from build123d import *

# Parameters (mm, degrees)
SKETCH_15_W          = 13
SKETCH_15_H          = 25
EXTRUDE_4_DEPTH      = 20
CUT_EXTRUDE_START    = 1
SKETCH_16_W          = 12
SKETCH_16_H          = 23
CUT_EXTRUDE_47_DEPTH = 24.6018292
CUT_EXTRUDE_48_DEPTH = 25.6018292


with BuildPart() as part:
    # 스케치15 → 보스-돌출4 (new body)
    with BuildSketch(Plane(origin=(0, 0, 0), x_dir=(1, 0, 0), z_dir=(0, 1, 0))):
        with Locations((0.5, 0)):
            Rectangle(SKETCH_15_W, SKETCH_15_H)
    extrude(amount=EXTRUDE_4_DEPTH)

    # 스케치16 → 컷-돌출47 (cut, through all)
    with BuildSketch(Plane(origin=(0, 0, 0), x_dir=(1, 0, 0), z_dir=(0, 1, 0)).offset(CUT_EXTRUDE_START)):
        Rectangle(SKETCH_16_W, SKETCH_16_H)
    extrude(amount=CUT_EXTRUDE_47_DEPTH, mode=Mode.SUBTRACT)

    # 스케치17 → 컷-돌출48 (cut, through all)
    with BuildSketch(Plane(origin=(0, 0, 0), x_dir=(1, 0, 0), z_dir=(0, 1, 0))):
        with BuildLine():
            Line((-6, -3.5), (6, -3.5))
            Line((6, -3.5), (6, 5.5))
            ThreePointArc((6, 5.5), (0, 11.5), (-6, 5.5))
            Line((-6, 5.5), (-6, -3.5))
        make_face()
    extrude(amount=CUT_EXTRUDE_48_DEPTH, mode=Mode.SUBTRACT)


solid = part.part
Check sheet for the modelled part. Datum: model origin and axes. Units: mm. A direction names the side the tool comes from. Round coordinates to 2 decimals unless told otherwise and drop trailing zeros. Loops run counter-clockwise (first coordinate to the right, second up) from the corner with the lowest first, then second, coordinate; pieces in that order, holes last. Notation, with made-up numbers: M 68,50.25 L 120,50.25 A20 cw 120,74.25 Z; hole C 67,68.25 d4. An arc over 180 degrees is marked long. One line per question, with ' | ' between items. Start each with the question number.
Item 1: Gauge pin test, flat ends, axial feed: pin 1 Ø4 at (x, z) = (2.5, -6) entering from +Y; pin 2 Ø3 at (x, z) = (-3, -9.5) entering from +Y; pin 3 Ø8 at (y, z) = (13, 4.5) entering from -X; pin 4 Ø3 at (x, z) = (-2, 8.5) entering from -Y. Record the tip position at first contact, or that the pin passes through.
Item 2: Section check A-A (y = 8). Record the boundary of the cut face in (x, z), and give its area (3 significant figures).
Item 3: Section check C-C (z = -4). Record the boundary of the cut face in (x, y), and give its area (3 significant figures).
Item 4: Set-up check for faces 5 (the face through (0, 10, 11.5)), 6 (the face through (6.2, 20, -0.1)), 7 (the face through (-0.1, 0.5, 3.5)): record each of +Z, -Z, +X, -X, +Y, -Y from which the full face is reachable in a straight line by a thin tool's end or side.
Item 5: Section check D-D (x = 2.75). Record the boundary of the cut face in (y, z), and give its area (3 significant figures).
Item 6: Release check for a two-part mould opening along X. For faces 1 (the face through (0.1, 0.5, -11.5)), 2 (the face through (7, 10, 0)), 3 (the face through (-6, 8, 12)), 4 (the face through (0, 10, -11.5)) record: released by +X, released by -X, zero draft, split by the parting line, or undercut.
Item 7: Scan lines: probe 1 along Z at (x, y) = (2.75, 17); probe 2 along X at (y, z) = (18.25, -9.5); probe 3 along Y at (x, z) = (-3, 4). Record each from-to range of solid material in increasing order.
Item 8: Section check B-B (x = 4.5). Record the boundary of the cut face in (y, z).
Worked out:
1) pin 1: through | pin 2: y = 1 | pin 3: x = 6 | pin 4: y = 0
2) outline: M -6,-12.5 L 7,-12.5 L 7,12.5 L -6,12.5 L -6,11.5 L 6,11.5 L 6,-11.5 L -6,-11.5 Z | area: 49.0 mm^2
3) outline: M 6,0 L 7,0 L 7,20 L 6,20 Z | area: 20.0 mm^2
4) face 5: -X, +Y | face 6: +Z, -Z, +X, -X, +Y | face 7: -X, +Y, -Y
5) outline: M 0,-12.5 L 20,-12.5 L 20,-11.5 L 1,-11.5 L 1,-10.83 L 0,-10.83 Z; M 0,3.5 L 1,3.5 L 1,11.5 L 20,11.5 L 20,12.5 L 0,12.5 Z | area: 48.7 mm^2
6) face 1: undercut | face 2: released by +X | face 3: released by -X | face 4: zero draft
7) probe 1: -12.5 to -11.5, 11.5 to 12.5 | probe 2: 6 to 7 | probe 3: 0 to 1
8) outline: M 0,-12.5 L 20,-12.5 L 20,-11.5 L 1,-11.5 L 1,-9.47 L 0,-9.47 Z; M 0,3.5 L 1,3.5 L 1,11.5 L 20,11.5 L 20,12.5 L 0,12.5 Z
